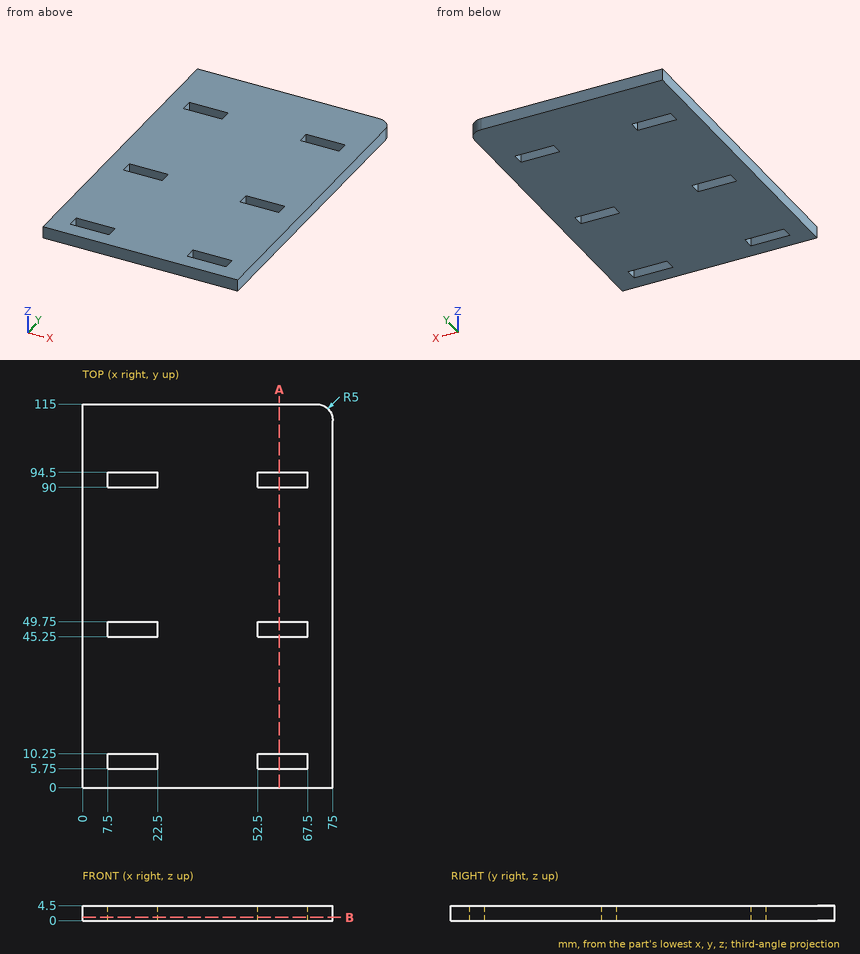
Check sheet for the drawn part. Datum: minimum x, y, z corner. Units: mm. Round coordinates to 2 decimals unless told otherwise and drop trailing zeros. Order: outer loops, then holes, each group sorted by start corner. A loop starts at its lowest first (then second) coordinate and runs counter-clockwise, first axis right, second up.
1. Thickness scan on L1, parallel to Y at x = 66.5, z = 3.8; L2, parallel to X at y = 49, z = 0.25; L3, parallel to Y at x = 70.5, z = 1.45. Record the ranges inside material, lowest first.
Final values:
L1: y = 0 to 5.75, 10.25 to 45.25, 49.75 to 90, 94.5 to 115
L2: x = 0 to 7.5, 22.5 to 52.5, 67.5 to 75
L3: y = 0 to 114.97
2. Section check A-A on x = 59. Record the cut outline in (y, z).
Final values:
outline: (0, 0) - (5.75, 0) - (5.75, 4.5) - (0, 4.5) - close; (10.25, 0) - (45.25, 0) - (45.25, 4.5) - (10.25, 4.5) - close; (49.75, 0) - (90, 0) - (90, 4.5) - (49.75, 4.5) - close; (94.5, 0) - (115, 0) - (115, 4.5) - (94.5, 4.5) - close
3. Section check B-B on z = 1. State how many separate pieces and enclosed holes the cut face has, then the cut area to 3 significant figures.
Final values:
separate pieces: 1
enclosed holes: 6
area: 8,210 mm2
